```python
from build123d import *

# Parameters (mm, degrees)
F0_W     = 120
F0_H     = 114
F0_R     = 1.75
F1_DEPTH = 6
F2_R     = 6
F3_R     = 4


with BuildPart() as f1:
    # F0 (on Top) → F1 (new body)
    with BuildSketch(Plane.XY):
        with Locations((0, 3)):
            Rectangle(F0_W, F0_H)
        with Locations((-56, -50)):
            Circle(F0_R, mode=Mode.SUBTRACT)
        with Locations((56, -50)):
            Circle(F0_R, mode=Mode.SUBTRACT)
        with Locations((0, 56)):
            Circle(F0_R, mode=Mode.SUBTRACT)
    extrude(amount=F1_DEPTH)

    # F2
    f2_edges = [f1.edges().sort_by_distance(p)[0] for p in [
        (-60, 60, 3),
        (60, 60, 3),
    ]]
    fillet(f2_edges, radius=F2_R)

    # F3
    f3_edges = [f1.edges().sort_by_distance(p)[0] for p in [
        (-60, -54, 3),
        (60, -54, 3),
    ]]
    fillet(f3_edges, radius=F3_R)


solid = f1.part
```
Source: CAD feature listing. Evaluate the final solid. Frame: model axes, mm. Give positions to 0.01 mm unless a question says otherwise; leave off trailing zeros. Loops run counter-clockwise (first coordinate to the right, second up) from the corner with the lowest first, then second, coordinate; pieces in that order, holes last. Notation, with made-up numbers: (41.5, -4) -> (85.5, -4) arc R18 cw to (85.5, 7) -> close; hole circle Ø5 at (61, -19). An arc over 180 degrees is marked (long way). Put each result on its own line as item: value. Start each with the question number.
1) Material intervals for probe 1 along Y at (x, z) = (0, 2.6); probe 2 along Y at (x, z) = (56, 2.45), sorted ascending.
2) Cut plane A-A (x = 0). Return loops of the section in (y, z), then the cut area to 3 significant figures.
3) Contact query for a flat-ended pin moving along its axis: P1, Ø3, axis at x = 0, y = 56, coming from the -Z side. Output: stop coordinate, or through.
4) Draft query along X for faces 1 (the face through (-58.289, 58.196, 3.042)), 2 (the face through (57.617, -50.67, 2.958)), 3 (the face through (-1, 60, 3)), 4 (the face through (-54.383, -50.67, 2.958)). Return one class per face: released by +X, released by -X, zero draft, split by the parting line, or undercut.
Results are:
1. probe 1: y = -54 to 54.25, 57.75 to 60
1. probe 2: y = -54 to -51.75, -48.25 to 59.66
2. outline: (-54, 0) -> (54.25, 0) -> (54.25, 6) -> (-54, 6) -> close; (57.75, 0) -> (60, 0) -> (60, 6) -> (57.75, 6) -> close
2. area: 663 mm2
3. P1: passes through
4. face 1: released by -X
4. face 2: undercut
4. face 3: zero draft
4. face 4: undercut
